```python
from build123d import *

# Parameters (mm, degrees)
RESSALTO_EXTRUS_O1_DEPTH   = 22
ESBO_O2_R                  = 10.5
ESBO_O2_R_2                = 7.5
RESSALTO_EXTRUS_O2_DEPTH   = 6.5
CHANFRO1_SIZE              = 0.8
CHANFRO2_SIZE              = 1.2
RESSALTO_EXTRUS_O3_START   = -1
ESBO_O3_R                  = 7.5
RESSALTO_EXTRUS_O3_DEPTH   = 1
ESBO_O4_R                  = 1.5
CORTE_EXTRUS_O1_DEPTH      = 18
ESBO_O5_R                  = 8
RESSALTO_EXTRUS_O4_DEPTH   = 3
FILETE2_R                  = 0.5
ESBO_O6_W                  = 42
ESBO_O6_H                  = 50
RESSALTO_EXTRUS_O5_DEPTH   = 15.25
FILETE3_R                  = 2
CORTE_EXTRUS_O2_DEPTH      = 19
CORTE_EXTRUS_O2_DEPTH_BACK = 70.25
CORTE_EXTRUS_O3_DEPTH      = 36
CORTE_EXTRUS_O3_DEPTH_BACK = 34.25
ESBO_O8_R                  = 3.575
ESBO_O9_R                  = 3.575
RESSALTO_EXTRUS_O6_DEPTH   = 10.85
ESBO_O10_R                 = 3.5
CORTE_EXTRUS_O4_DEPTH      = 5.7
ESBO_O13_R                 = 2
RESSALTO_EXTRUS_O7_DEPTH   = 10


with BuildPart() as part:
    # Esbo_o1 → Ressalto-extrus_o1 (new body)
    with BuildSketch(Plane.XY):
        with BuildLine():
            Line((-31.85, 15.65), (31.85, 15.65))
            ThreePointArc((31.85, 15.65), (47.5, 0), (31.85, -15.65))
            Line((31.85, -15.65), (-31.85, -15.65))
            ThreePointArc((-31.85, -15.65), (-47.5, 0), (-31.85, 15.65))
        make_face()
    extrude(amount=RESSALTO_EXTRUS_O1_DEPTH)

    # Esbo_o2 → Ressalto-extrus_o2 (add)
    with BuildSketch(Plane.XY.offset(22)):
        with Locations(Location((0, 0, 0), (0, 0, 180))):
            Circle(ESBO_O2_R)
        with Locations(Location((0, 0, 0), (0, 0, 180))):
            Circle(ESBO_O2_R_2, mode=Mode.SUBTRACT)
    extrude(amount=RESSALTO_EXTRUS_O2_DEPTH)

    # Chanfro1
    chanfro1_edges = [part.edges().sort_by_distance(p)[0] for p in [
        (10.5, 0, 28.5),
        (7.5, 0, 28.5),
    ]]
    chamfer(chanfro1_edges, length=CHANFRO1_SIZE)

    # Chanfro2
    chanfro2_edges = [part.edges().sort_by_distance(p)[0] for p in [
        (10.5, 0, 22),
    ]]
    chamfer(chanfro2_edges, length=CHANFRO2_SIZE)

    # Esbo_o3 → Ressalto-extrus_o3 (add)
    with BuildSketch(Plane.XY.offset(27.7).offset(RESSALTO_EXTRUS_O3_START)):
        with Locations(Location((0, 0, 0), (0, 0, 180))):
            Circle(ESBO_O3_R)
    extrude(amount=RESSALTO_EXTRUS_O3_DEPTH)

    # Esbo_o4 → Corte-extrus_o1 (cut)
    with BuildSketch(Plane.XY.offset(22)):
        with Locations((26.2, 0)):
            Circle(ESBO_O4_R)
    extrude(amount=-CORTE_EXTRUS_O1_DEPTH, mode=Mode.SUBTRACT)

    # Esbo_o5 → Ressalto-extrus_o4 (add)
    with BuildSketch(Plane.XZ.offset(15.65)):
        with Locations(Location((0, 11, 0), (0, 0, 90))):
            Circle(ESBO_O5_R)
    extrude(amount=RESSALTO_EXTRUS_O4_DEPTH)

    # Filete2
    filete2_edges = [part.edges().sort_by_distance(p)[0] for p in [
        (0, -15.65, 3),
        (0, -18.65, 3),
        (0, 15.65, 0),
        (47.5, 0, 0),
        (0, -15.65, 0),
        (-47.5, 0, 0),
    ]]
    fillet(filete2_edges, radius=FILETE2_R)



with BuildPart() as body_2:
    # Esbo_o6 → Ressalto-extrus_o5 (new body)
    with BuildSketch(Plane(origin=(0, -21.15, 0), x_dir=(-1, 0, 0), z_dir=(0, -1, 0))):
        with Locations((0, 5)):
            Rectangle(ESBO_O6_W, ESBO_O6_H)
    extrude(amount=RESSALTO_EXTRUS_O5_DEPTH)

    # Filete3
    filete3_edges = [body_2.edges().sort_by_distance(p)[0] for p in [
        (-21, -36.4, -5),
        (21, -36.4, -5),
        (-21, -21.15, -5),
        (21, -21.15, -5),
    ]]
    fillet(filete3_edges, radius=FILETE3_R)

    # Esbo_o7 → Corte-extrus_o2 (cut, two sides: drawn at the far end of the back side and taken through both)
    with BuildSketch(Plane.ZY.offset(21).offset(-CORTE_EXTRUS_O2_DEPTH_BACK)):
        with BuildLine():
            Line((-30, -26.65), (16.5, -26.65))
            Line((16.5, -26.65), (16.5, -38.046721954))
            Line((16.5, -38.046721954), (15.730351624, -38.046721954))
            Line((15.730351624, -38.046721954), (15.730351624, -33.8624466))
            ThreePointArc((15.730351624, -33.8624466), (13.826545702, -29.266252522), (9.230351624, -27.3624466))
            Line((9.230351624, -27.3624466), (-30, -27.3624466))
            Line((-30, -27.3624466), (-31.616650622, -27.3624466))
            Line((-31.616650622, -27.3624466), (-31.616650622, -26.65))
            Line((-31.616650622, -26.65), (-30, -26.65))
        make_face()
    extrude(amount=CORTE_EXTRUS_O2_DEPTH + CORTE_EXTRUS_O2_DEPTH_BACK, mode=Mode.SUBTRACT)


with BuildPart() as corte_extrus_o2_piece_1:
    # of the separate pieces the step leaves, piece 1, a body of its own (corte_extrus_o2_pieces)
    add(body_2.part.solids().sort_by_distance((-21, -27.3624466, -30))[0])


with BuildPart() as corte_extrus_o2_piece_2:
    # of the separate pieces the step leaves, piece 2, a body of its own (corte_extrus_o2_pieces)
    add(body_2.part.solids().sort_by_distance((-21, -23.15, 20))[0])


with BuildPart() as corte_extrus_o3_tool:
    # Esbo_o8 → Corte-extrus_o3 (new, two sides: drawn at the far end of the back side and taken through both)
    with BuildSketch(Plane(origin=(0, 0, 0), x_dir=(0, 0, -1), z_dir=(1, 0, 0)).offset(-CORTE_EXTRUS_O3_DEPTH_BACK)):
        with Locations((30, -27.0062233)):
            Circle(ESBO_O8_R)
    extrude(amount=CORTE_EXTRUS_O3_DEPTH + CORTE_EXTRUS_O3_DEPTH_BACK)


with BuildPart() as corte_extrus_o2_piece_1_1:
    add(corte_extrus_o2_piece_1.part)

    # Corte-extrus_o3: cut by corte_extrus_o3_tool
    add(corte_extrus_o3_tool.part, mode=Mode.SUBTRACT)



with BuildPart() as corte_extrus_o2_piece_2_1:
    add(corte_extrus_o2_piece_2.part)

    # Corte-extrus_o3: cut by corte_extrus_o3_tool
    add(corte_extrus_o3_tool.part, mode=Mode.SUBTRACT)


with BuildPart() as corte_extrus_o2_piece_1_2:
    add(corte_extrus_o2_piece_1_1.part)

    add(corte_extrus_o2_piece_2_1.part)  # Ressalto-extrus_o6 merges Corte-extrus_o2 piece 2
    # Esbo_o9 → Ressalto-extrus_o6 (add, symmetric)
    with BuildSketch(Plane(origin=(0, 0, 0), x_dir=(0, 0, -1), z_dir=(1, 0, 0))):
        with Locations((30, -27.0062233)):
            Circle(ESBO_O9_R)
    extrude(amount=RESSALTO_EXTRUS_O6_DEPTH, both=True)

    # Esbo_o10 → Corte-extrus_o4 (cut)
    with BuildSketch(Plane.XZ.offset(36.4)):
        with Locations(Location((0, -7.134824188, 0), (0, 0, 270))):
            Circle(ESBO_O10_R)
    extrude(amount=-CORTE_EXTRUS_O4_DEPTH, mode=Mode.SUBTRACT)


with BuildPart() as part_1:
    add(part.part)

    add(corte_extrus_o2_piece_1_2.part)  # Revolu_o1 merges Corte-extrus_o2 piece 1
    # Esbo_o12 → Revolu_o1 (revolve)
    with BuildSketch(Plane.XY.offset(11), mode=Mode.PRIVATE) as revolu_o1_sk:
        with BuildLine():
            Line((0, -15.65), (0, -21.15))
            Line((0, -21.15), (-8, -21.15))
            ThreePointArc((-8, -21.15), (-4.85412196, -17.157640786), (0, -15.65))
        make_face()
    revolve(revolu_o1_sk.sketch.rotate(Axis((0, -15.65, 11), (0, -1, 0)), 90), axis=Axis((0, -15.65, 11), (0, -1, 0)))

    # Esbo_o13 → Ressalto-extrus_o7 (add)
    with BuildSketch(Plane(origin=(0, 0, 0), x_dir=(-1, 0, 0), z_dir=(0, 0, -1))):
        with Locations(Location((-26.85, -7.65, 0), (0, 0, 180))):
            Circle(ESBO_O13_R)
    extrude(amount=RESSALTO_EXTRUS_O7_DEPTH)


solid = part_1.part
```
The model under review builds one solid part; all positions refer to its coordinate system, in mm. A direction names the side the tool comes from. Coordinates: 2 decimals unless noted, no trailing zeros. Write each loop counter-clockwise with the first axis right and the second up, starting at its lowest first coordinate (ties: lowest second). Pieces come first, ordered by that corner, then holes.
1) Machinability: for faces 1 (the face through (0, -33, -30)), 2 (the face through (28.758, -8.251, -4.93)), 3 (the face through (0, -29, 20)), which of the approach directions +Z, -Z, +X, -X, +Y, -Y give a long, thin tool a straight path to every point of the face, cutting with its end or side? Answer none if there is none.
2) To check wall thickness, follow probe 1 along Y at (x, z) = (0, 25); probe 2 along Z at (x, y) = (-1, 7); probe 3 along Y at (x, z) = (2, -13.5). State the ranges of each line that lie inside material, in increasing order.
3) The part is to be moulded in two halves that separate along Z. For faces 4 (the face through (0, 0, 26.7)), 5 (the face through (-21, -31, -7)), 6 (the face through (-4.032, -6.324, 24.317)), 7 (the face through (0, -22, -30)), say which applies: pulls with the +Z half, pulls with the -Z half, needs draft (parallel to the pull), parting line crosses it, or undercut.
4) We need section A-A on z = -24.5. State the section outline as (x, y) points.
5) Clearance check with flat-ended pins moving along their axes: pin 1 Ø6 at (x, y) = (8, -16) entering from -Z; pin 2 Ø7.5 at (x, y) = (0.5, 0) entering from +Z; pin 3 Ø2.5 at (x, y) = (3.5, -22.5) entering from -Z. State where each tip first meets the part, or that it passes through.
6) We need section B-B on x = -17. State the section outline as (y, z) points (3 decimals).
7) We need section C-C on z = 11. Count the separate pieces of the cut face and the enclosed holes in it, then the cut area to 3 significant figures.
8) We need section D-D on z = 24.5. State the section outline as (x, y) points.
Answer list:
1. face 1: -Z, +X, -X, -Y
1. face 2: -Z
1. face 3: +Z, +X, -X, -Y
2. probe 1: y = -10.5 to -7.5, 7.5 to 10.5
2. probe 2: z = 0 to 22, 26.7 to 27.7
2. probe 3: y = -36.4 to -27.36, -26.65 to -21.15
3. face 4: undercut
3. face 5: needs draft
3. face 6: undercut
3. face 7: pulls with the -Z half
4. outline: (-21, -34.4) arc R2 ccw to (-19, -36.4) - (19, -36.4) arc R2 ccw to (21, -34.4) - (21, -27.36) - (-21, -27.36) - close; (-21, -26.65) - (21, -26.65) - (21, -23.15) arc R2 ccw to (19, -21.15) - (-19, -21.15) arc R2 ccw to (-21, -23.15) - close
5. pin 1: stops at z = 0
5. pin 2: stops at z = 27.7
5. pin 3: stops at z = -31.48
6. outline: (-36.4, -30) - (-30.581, -30) arc R3.575 cw to (-27.362, -26.443) - (-27.362, 9.23) arc R6.5 ccw to (-33.862, 15.73) - (-36.4, 15.73) - close; (-36.4, 16.5) - (-26.65, 16.5) - (-26.65, -26.443) arc R3.575 cw to (-23.431, -30) - (-21.15, -30) - (-21.15, 20) - (-36.4, 20) - close; (-15.65, 0.5) arc R0.5 ccw to (-15.15, 0) - (15.15, 0) arc R0.5 ccw to (15.65, 0.5) - (15.65, 22) - (-15.65, 22) - close
7. separate pieces: 2
7. enclosed holes: 1
7. area: 3,440 mm2
8. outline: circle Ø21 at (0, 0); hole circle Ø15 at (0, 0)
